```python
from build123d import *

# Parameters (mm, degrees)
CUT_EXTRUDE1_DEPTH = 3.6195


with BuildPart() as part:
    # Sketch2 → Revolve1 (revolve)
    with BuildSketch(Plane(origin=(0, 0, 0), x_dir=(0, 0, -1), z_dir=(1, 0, 0)), mode=Mode.PRIVATE) as revolve1_sk:
        Polygon((-15.1384, 0), (24.6126, 0), (24.6126, 1.894416667), (24.094016667, 2.413), (-10.3124, 2.413), (-10.3124, 3.450166667), (-10.830983333, 3.96875), (-14.619816667, 3.96875), (-15.1384, 3.450166667), align=None)
    revolve(revolve1_sk.sketch.rotate(Axis((0, 0, 10.3124), (0, 0, -1)), 180), axis=Axis((0, 0, 10.3124), (0, 0, -1)))

    # Sketch3 → Cut-Extrude1 (cut)
    with BuildSketch(Plane.XY.offset(15.1384)):
        Polygon((1.14567944, 1.984375), (-1.14567944, 1.984375), (-2.291358881, 0), (-1.14567944, -1.984375), (1.14567944, -1.984375), (2.291358881, 0), align=None)
    extrude(amount=-CUT_EXTRUDE1_DEPTH, mode=Mode.SUBTRACT)

    # Cut-Extrude2 cone 1 section (on through the dimple's axis) → Cut-Extrude2 (revolve, cut)
    with BuildSketch(Plane(origin=(0, 0, 15.1384), x_dir=(0, -1, 0), z_dir=(1, 0, 0))):
        Polygon((0, 0), (2.291358881, 0), (0, 2.291358881), align=None)
    revolve(axis=Axis((0, 0, 15.1384), (0, 0, -1)), mode=Mode.SUBTRACT)


solid = part.part
```
Geometry: final body of the model. Coordinates: model frame, mm. A direction names the side the tool comes from. Round coordinates to 2 decimals unless told otherwise and drop trailing zeros. Order: outer loops, then holes, each group sorted by start corner. A loop starts at its lowest first (then second) coordinate and runs counter-clockwise, first axis right, second up. Notation, with made-up numbers: (24.5, -29.75) - (58.5, -29.75) arc R18 ccw to (58.5, -19.75) - close; hole circle Ø6 at (-32.75, 20.5). An arc over 180 degrees is marked (long way). Write item = value, one per line. Start each with the question number.
Q1. Pull-direction query (X, two-part tool) for faces 3 (the flat face through (0, 0, -24.613)), 4 (the conical face through (1.857, -1.054, 14.983)), 5 (the cylindrical face through (3.874, 0.86, 12.752)); classes: +X half, -X half, draft (parallel to the pull), parting line (faces both ways), or undercut.
Q2. Pin query (flat end, axial travel): pin 1 (4 mm diameter, centred on y = -1, z = -13.5, fed in from +X); pin 2 (1 mm diameter, centred on y = -2, z = 10.5, fed in from +X); pin 3 (1.5 mm diameter, centred on y = 1.5, z = 1, fed in from +X). Return the tip coordinate at first contact, or that it passes through.
Q3. Ray query, line 1 (Y direction, x = -1.5, z = 0.5); line 2 (Z direction, x = 2.5, y = 2); line 3 (X direction, y = 1.25, z = 12). Return the intervals inside material, ascending. Write a range as from..to.
Q4. Cut plane B-B on z = -5. Return the cut outline in (x, y), and give its area (3 significant figures).
Q5. Cut plane A-A on x = 0. Return the cut outline in (y, z), and give its area (3 significant figures).
Q6. Access query for faces 1 (the cylindrical face through (1.468, 1.915, -6.65)), 2 (the flat face through (-1.71, 1.01, 13.35)). Directions: +Z, -Z, +X, -X, +Y, -Y. A direction counts if a zero-diameter tool reaches every point of the face in a straight line with its end or side. Return the directions, or none.
Outcome:
q1.face_3 = draft
q1.face_4 = undercut
q1.face_5 = parting line
q2.pin_1 = 2.41
q2.pin_2 = 3.62
q2.pin_3 = 2.29
q3.line_1 = -1.89..1.89
q3.line_2 = 10.31..15.14
q3.line_3 = -3.77..-1.57, 1.57..3.77
q4.outline = circle Ø4.83 at (0, 0)
q4.area = 18.3 mm^2
q5.outline = (-3.97, 10.83) - (-3.45, 10.31) - (-2.41, 10.31) - (-2.41, -24.09) - (-1.89, -24.61) - (1.89, -24.61) - (2.41, -24.09) - (2.41, 10.31) - (3.45, 10.31) - (3.97, 10.83) - (3.97, 14.62) - (3.45, 15.14) - (2.29, 15.14) - (1.98, 14.83) - (1.98, 11.52) - (-1.98, 11.52) - (-1.98, 14.83) - (-2.29, 15.14) - (-3.45, 15.14) - (-3.97, 14.62) - close
q5.area = 192 mm^2
q6.face_1 = -Z
q6.face_2 = +Z
